```python
from build123d import *

# Parameters (mm, degrees)
SKETCH1_R                       = 50.8
SKETCH1_R_2                     = 47.625
BOSS_EXTRUDE1_DEPTH             = 19.05
SKETCH5_W                       = 2.5527
SKETCH5_H                       = 82.55
TAP_DRILL_FOR_1_4_20_TAP2_D     = 5.1054
TAP_DRILL_FOR_1_4_20_TAP2_DEPTH = 82.55
SKETCH10_R                      = 1.905
CUT_EXTRUDE3_DEPTH              = 83.5500001
CUT_EXTRUDE3_DEPTH_BACK         = 20.0500001


with BuildPart() as part:
    # Sketch1 → Boss-Extrude1 (new body)
    with BuildSketch(Plane(origin=(0, 0, 0), x_dir=(1, 0, 0), z_dir=(0, 1, 0))):
        Circle(SKETCH1_R)
        Circle(SKETCH1_R_2, mode=Mode.SUBTRACT)
    extrude(amount=BOSS_EXTRUDE1_DEPTH)

    # Sketch5 → Tap Drill for 1/4-20 Tap1 (revolve, cut)
    with BuildSketch(Plane(origin=(0, 9.525, 31.75), x_dir=(0, -1, 0), z_dir=(1, 0, 0))):
        with Locations((1.27635, 41.275)):
            Rectangle(SKETCH5_W, SKETCH5_H)
    revolve(axis=Axis((0, 9.525, 38.1), (0, 0, -1)), mode=Mode.SUBTRACT)

    # Tap Drill for 1/4-20 Tap2
    with Locations(Plane(origin=(0, 0, -31.75), x_dir=(1, 0, 0), z_dir=(0, 0, -1))):
        with Locations((0, -9.525)):
            Hole(TAP_DRILL_FOR_1_4_20_TAP2_D / 2, depth=TAP_DRILL_FOR_1_4_20_TAP2_DEPTH)

    # Sketch10 → Cut-Extrude3 (cut, two sides)
    with BuildSketch(Plane(origin=(-31.75, 0, 0), x_dir=(0, 0, -1), z_dir=(1, 0, 0))) as cut_extrude3_sk:
        with Locations((0, 9.487883811)):
            Circle(SKETCH10_R)
    extrude(amount=CUT_EXTRUDE3_DEPTH, mode=Mode.SUBTRACT)
    extrude(cut_extrude3_sk.sketch, amount=-CUT_EXTRUDE3_DEPTH_BACK, mode=Mode.SUBTRACT)


solid = part.part
```
The listing builds one solid part. Answer for the finished solid, in the listing's coordinates (mm). Coordinates: 2 decimals unless noted, no trailing zeros. Write each loop counter-clockwise with the first axis right and the second up, starting at its lowest first coordinate (ties: lowest second). Pieces come first, ordered by that corner, then holes. Notation, with made-up numbers: (81, -31.5) - (92, -31.5) arc R6 ccw to (92, -25.5) - close; hole circle Ø5 at (-23, 4.5). An arc over 180 degrees is marked (long way). Return JSON: item names as keys, results as strings. Group by question number.
1. Straight lines are drawn through the part: L1, parallel to X at y = 7, z = 0 (3 decimals); L2, parallel to Y at x = 0, z = 50; L3, parallel to Y at x = 50, z = 0. For each, find the intervals that lie inside material, in ascending order.
2. Determine the mould class of faces 1 (the cylindrical face through (0.553, 12.017, 49.201)), 2 (the flat face through (-15.3, 19.05, -45.4)), 3 (the flat face through (-15.3, 0, -45.4)) for opening direction Y: released by +Y, released by -Y, zero draft, split by the parting line, or undercut.
3. A cutting plane is placed at D-D, the plane x = 42.5. Determine the outline of the cut face in (y, z), plus the area to 3 significant figures.
4. Given pin 1 (1.5 mm diameter, centred on y = 4, z = 31, fed in from -X); pin 2 (4 mm diameter, centred on y = 3.5, z = 29.5, fed in from -X); pin 3 (8 mm diameter, centred on x = 0, y = 9.525, fed in from -Z); pin 4 (1.5 mm diameter, centred on y = 12.5, z = -10, fed in from +X), each flat-ended and moving along its own axis, determine where each tip first touches the part or whether it passes through.
5. A cutting plane is placed at B-B, the plane x = 0. Determine the outline of the cut face in (y, z) (3 decimals).
6. A cutting plane is placed at C-C, the plane z = 32.5. Determine the outline of the cut face in (x, y).
7. A cutting plane is placed at A-A, the plane z = 0. Determine the outline of the cut face in (x, y) (3 decimals).
Ans:
{
 "1": {"L1": "-50.8 to -47.625, 47.625 to 50.8", "L2": "0 to 6.97, 12.08 to 19.05", "L3": "0 to 7.58, 11.39 to 19.05"},
 "2": {"face 1": "undercut", "face 2": "released by +Y", "face 3": "released by -Y"},
 "3": {"outline": "(0, -27.83) - (19.05, -27.83) - (19.05, -21.49) - (0, -21.49) - close; (0, 21.49) - (19.05, 21.49) - (19.05, 27.83) - (0, 27.83) - close", "area": "241 mm²"},
 "4": {"pin 1": "x = -40.81", "pin 2": "x = -42.71", "pin 3": "z = -50.8", "pin 4": "x = 49.95"},
 "5": {"outline": "(0, -50.8) - (6.972, -50.8) - (6.972, -47.625) - (0, -47.625) - close; (0, 47.625) - (6.972, 47.625) - (6.972, 50.8) - (0, 50.8) - close; (12.078, -50.8) - (19.05, -50.8) - (19.05, -47.625) - (12.078, -47.625) - close; (12.078, 47.625) - (19.05, 47.625) - (19.05, 50.8) - (12.078, 50.8) - close"},
 "6": {"outline": "(-39.04, 0) - (-34.81, 0) - (-34.81, 19.05) - (-39.04, 19.05) - close; (34.81, 0) - (39.04, 0) - (39.04, 19.05) - (34.81, 19.05) - close"},
 "7": {"outline": "(-50.8, 0) - (-47.625, 0) - (-47.625, 7.583) - (-50.8, 7.583) - close; (-50.8, 11.393) - (-47.625, 11.393) - (-47.625, 19.05) - (-50.8, 19.05) - close; (47.625, 0) - (50.8, 0) - (50.8, 7.583) - (47.625, 7.583) - close; (47.625, 11.393) - (50.8, 11.393) - (50.8, 19.05) - (47.625, 19.05) - close"}
}
